Verification items for the finished model (mm, model axes). Face numbers are marked on the shaded views. Round coordinates to 2 decimals unless told otherwise and drop trailing zeros. Order: outer loops, then holes, each group sorted by start corner. A loop starts at its lowest first (then second) coordinate and runs counter-clockwise, first axis right, second up. Notation, with made-up numbers: (4, 63.5) -> (17, 63.5) arc R22 ccw to (17, 85.5) -> close; hole circle Ø2 at (-23, 60.25). An arc over 180 degrees is marked (long way). Return JSON: item names as keys, results as strings. Group by question number.
Item 1: Depth check by flat-ended pin: pin 1 Ø1.5 at (x, y) = (-50.5, 30.5) entering from +Z. Enter the tip coordinate at first touch or a pass-through.
Item 2: Draft check along X on the marked faces 1, 2 and 3. Enter one of: pulls with the +X half, pulls with the -X half, needs draft (parallel to the pull), parting line crosses it, or undercut.
Item 3: Scan lines: probe 1 along X at (y, z) = (43.5, -58.5); probe 2 along X at (y, z) = (29, -37); probe 3 along Z at (x, y) = (-346, 46). Record each from-to range of solid material in increasing order. Write a range as from..to.
Item 4: Sectioned sample at A-A on z = -17.5. Record the cut outline in (x, y).
Item 5: Sectioned sample at B-B on z = -81.5. Record the cut outline in (x, y).
Item 6: Sectioned sample at D-D on x = -146.5. Record the cut outline in (y, z).
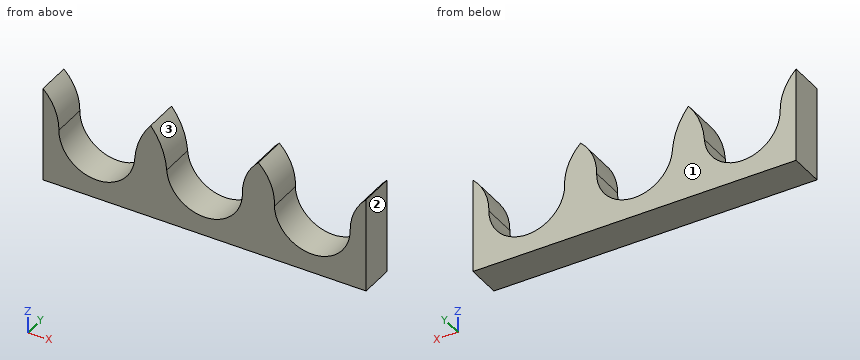
Autodesk Inventor part; units mm, degrees
ref_plane "YZ Plane" through (0, 0, 0) normal (1, 0, 0) x (0, 1, 0)
ref_plane "XZ Plane" through (0, 0, 0) normal (0, 1, 0) x (-1, 0, 0)
ref_plane "XY Plane" through (0, 0, 0) normal (0, 0, 1) x (1, 0, 0)
sketch "Sketch1" plane through (0, 0, 0) normal (0, 0, 1) x (1, 0, 0)
  line L0 (0, 0) -> (-476.25, 0)
  line L1 (-476.25, 0) -> (-476.25, 50.8)
  line L2 (-476.25, 50.8) -> (0, 50.8)
  line L3 (0, 50.8) -> (0, 0)
  dimension "d5" = 50.8
  dimension "d6" = 476.25
extrude "Extrusion1" add sketch "Sketch1" against normal blind 139.7
sketch "Sketch2" plane through (-476.25, 50.8, 0) normal (0, 1, 0) x (1, 0, 0)
  line L0 (0, 0) -> (476.25, 0)
  circle A0 centre (396.875, 55.88) radius 55.88
  arc A1 (452.7532, 55.4333) -> (476.25, 0) centre (528.4627, 54.8281) ccw
  line L1 (476.25, 139.7) -> (0, 139.7)
  line L2 (476.25, 0) -> (476.25, 139.7)
  line L3 (158.75, 139.7) -> (158.75, 0)
  line L4 (317.5, 139.7) -> (317.5, 0)
  circle A2 centre (238.125, 55.88) radius 55.88
  circle A3 centre (79.375, 55.88) radius 55.88
  arc A4 (317.5, 0) -> (341.0467, 58.2841) centre (268.3126, 53.7701) ccw
  arc A5 (135.1205, 59.7553) -> (158.75, 0) centre (241.1273, 67.1248) ccw
  arc A6 (0, 0) -> (23.4968, 55.4333) centre (-52.2127, 54.8281) ccw
  arc A7 (158.75, 0) -> (182.3795, 59.7553) centre (76.3727, 67.1248) ccw
  arc A8 (293.9963, 54.8959) -> (317.5, 0) centre (366.8591, 53.6126) ccw
  dimension "d9" = 111.76
  dimension "d10" = 55.88
  dimension "d11" = 79.375
  dimension "d14" = 158.75
  dimension "d15" = 158.75
  dimension "d16" = 79.375
  dimension "d17" = 79.375
extrude "Extrusion3" cut sketch "Sketch2" against normal blind 139.7 contours A6 A3 L0 | A7 A2 L0 | A3 A5 L0 | A3 | A2 A8 L0 | A2 | A4 A0 L0 | A0 A1 L0 | A0 A4 picked at (415.2449, 59.3205)
properties part number "swirvy for illustrator"
Recorded:
{
 "1": {"pin 1": "z = -103.26"},
 "2": {"face 1": "needs draft", "face 2": "pulls with the +X half", "face 3": "undercut"},
 "3": {"probe 1": "-476.25..-452.69, -341.03..-293.97, -182.31..-135.19, -23.56..0", "probe 2": "-476.25..-454.88, -337.03..-297.97, -180.35..-137.02, -21.37..0", "probe 3": "-139.7..-79"},
 "4": {"outline": "(-476.25, 0) -> (-462.59, 0) -> (-462.59, 50.8) -> (-476.25, 50.8) -> close; (-329.09, 0) -> (-305.91, 0) -> (-305.91, 50.8) -> (-329.09, 50.8) -> close; (-172.69, 0) -> (-144.73, 0) -> (-144.73, 50.8) -> (-172.69, 50.8) -> close; (-13.66, 0) -> (0, 0) -> (0, 50.8) -> (-13.66, 50.8) -> close"},
 "5": {"outline": "(-476.25, 0) -> (-446.54, 0) -> (-446.54, 50.8) -> (-476.25, 50.8) -> close; (-347.21, 0) -> (-287.79, 0) -> (-287.79, 50.8) -> (-347.21, 50.8) -> close; (-188.46, 0) -> (-129.04, 0) -> (-129.04, 50.8) -> (-188.46, 50.8) -> close; (-29.71, 0) -> (0, 0) -> (0, 50.8) -> (-29.71, 50.8) -> close"},
 "6": {"outline": "(0, -139.7) -> (50.8, -139.7) -> (50.8, -14.58) -> (0, -14.58) -> close"}
}
